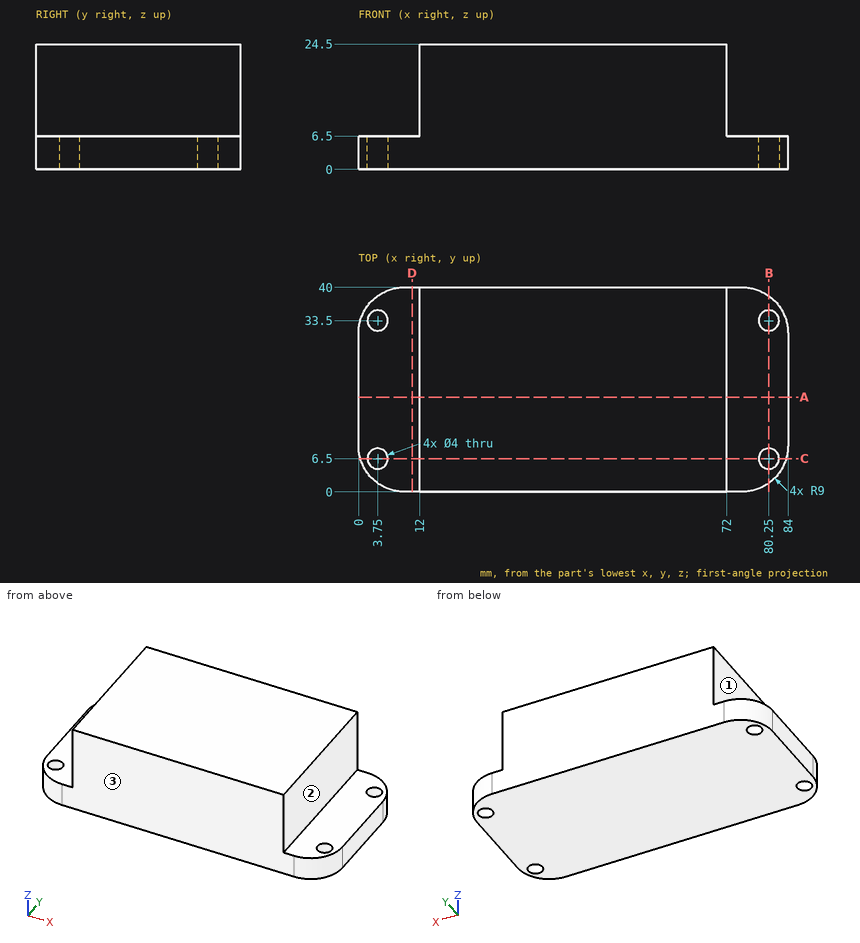
Part print with two shaded views. Sizes in mm from the minimum x, y, z corner. A direction names the side the tool comes from. Give positions to 0.01 mm unless a question says otherwise; leave off trailing zeros. Order: outer loops, then holes, each group sorted by start corner. A loop starts at its lowest first (then second) coordinate and runs counter-clockwise, first axis right, second up. Notation, with made-up numbers: M 69,32 L 114,32 A14 ccw 114,50 Z; hole C -23,56 d4. An arc over 180 degrees is marked long. Write item = value, one per line.
Q1. Cut at A-A, the plane y = 18.5. List the corners of the cut face in (x, z), then the cut area to 3 significant figures.
Derived:
outline = M 0,0 L 84,0 L 84,6.5 L 72,6.5 L 72,24.5 L 12,24.5 L 12,6.5 L 0,6.5 Z
area = 1,630 mm2
Q2. Cut at D-D, the plane x = 10.5. List the corners of the cut face in (y, z), then the cut area to 3 significant figures.
Derived:
outline = M 0,0 L 40,0 L 40,6.5 L 0,6.5 Z
area = 260 mm2
Q3. Flat gauge pins, fed straight in: pin 1 (3.5 mm diameter, centred on x = 79, y = 18.5, fed in from +Z); pin 2 (5 mm diameter, centred on x = 58, z = 17.5, fed in from -Y); pin 3 (2 mm diameter, centred on x = 9.5, z = 14.5, fed in from +Y); pin 4 (5 mm diameter, centred on y = 4, z = 10.5, fed in from -X). Where does each tip first touch, or does it go through?
Derived:
pin_1 = 6.5
pin_2 = 0
pin_3 = through
pin_4 = 12
Q4. Tool access for the marked faces 1, 2 and 3: list every direction of +Z, -Z, +X, -X, +Y, -Y with a clear straight run to the whole face (end or side of a thin tool).
Derived:
face_1 = +Z, -X, +Y, -Y
face_2 = +Z, +X, +Y, -Y
face_3 = +Z, -Z, +X, -X, -Y
Q5. Cut at B-B, the plane x = 80.25. List the corners of the cut face in (y, z).
Derived:
outline = M 1.69,0 L 4.5,0 L 4.5,6.5 L 1.69,6.5 Z; M 8.5,0 L 31.5,0 L 31.5,6.5 L 8.5,6.5 Z; M 35.5,0 L 38.31,0 L 38.31,6.5 L 35.5,6.5 Z
Q6. Drill centre lines: line 1 (Y direction, x = 3.75, z = 2.25); line 2 (X direction, y = 6.5, z = 4.25); line 3 (X direction, y = 9, z = 15.25). Where is each one in solid material? Low to high. Write a range as [from, to].
Derived:
line_1 = [1.69, 4.5], [8.5, 31.5], [35.5, 38.31]
line_2 = [0.35, 1.75], [5.75, 78.25], [82.25, 83.65]
line_3 = [12, 72]
Q7. Cut at C-C, the plane y = 6.5. List the corners of the cut face in (x, z).
Derived:
outline = M 0.35,0 L 1.75,0 L 1.75,6.5 L 0.35,6.5 Z; M 5.75,0 L 78.25,0 L 78.25,6.5 L 72,6.5 L 72,24.5 L 12,24.5 L 12,6.5 L 5.75,6.5 Z; M 82.25,0 L 83.65,0 L 83.65,6.5 L 82.25,6.5 Z
